```python
from build123d import *

# Parameters (mm, degrees)
SKETCH1_R               = 5
SKETCH1_W               = 4.1
SKETCH1_H               = 4.1
BOSS_EXTRUDE1_DEPTH     = 6
SKETCH1_3_R             = 8
SKETCH1_3_R_2           = 5
BOSS_EXTRUDE2_DEPTH     = 3
SKETCH1_6_R             = 8
SKETCH1_6_R_2           = 5
CUT_EXTRUDE_THIN1_DEPTH = 1.5


with BuildPart() as part:
    # Sketch1 → Boss-Extrude1 (new, symmetric)
    with BuildSketch(Plane.XY):
        Circle(SKETCH1_R)
        Rectangle(SKETCH1_W, SKETCH1_H, mode=Mode.SUBTRACT)
    extrude(amount=BOSS_EXTRUDE1_DEPTH, both=True)

    # Sketch1<3> → Boss-Extrude2 (add, symmetric)
    # profile 1 of 2: a face of its own
    with BuildSketch(Plane.XY):
        Circle(SKETCH1_3_R)
        Circle(SKETCH1_3_R_2, mode=Mode.SUBTRACT)
    # profile 2 of 2: a face of its own
    with BuildSketch(Plane.XY):
        Circle(SKETCH1_3_R)
        Circle(SKETCH1_3_R_2, mode=Mode.SUBTRACT)
    extrude(amount=BOSS_EXTRUDE2_DEPTH, both=True)

    # Sketch1<6> → Cut-Extrude-Thin1 (cut, symmetric)
    with BuildSketch(Plane.XY):
        Circle(SKETCH1_6_R)
        Circle(SKETCH1_6_R_2, mode=Mode.SUBTRACT)
    extrude(amount=CUT_EXTRUDE_THIN1_DEPTH, both=True, mode=Mode.SUBTRACT)


solid = part.part
```
The listing builds one solid part. Answer for the finished solid, in the listing's coordinates (mm). A direction names the side the tool comes from. Coordinates: 2 decimals unless noted, no trailing zeros. Loops run counter-clockwise (first coordinate to the right, second up) from the corner with the lowest first, then second, coordinate; pieces in that order, holes last. Notation, with made-up numbers: (-35, 16.25) - (-14, 16.25) arc R26 cw to (-14, 52.25) - close; hole circle Ø7 at (15.25, -28). An arc over 180 degrees is marked (long way). Write item = value, one per line.
1) Section D-D (x = 2.5) is taken. Determine the outline of the cut face in (y, z), plus the area to 3 significant figures.
Responses:
outline = (-7.6, -3) - (-4.33, -3) - (-4.33, -6) - (4.33, -6) - (4.33, -3) - (7.6, -3) - (7.6, -1.5) - (4.33, -1.5) - (4.33, 1.5) - (7.6, 1.5) - (7.6, 3) - (4.33, 3) - (4.33, 6) - (-4.33, 6) - (-4.33, 3) - (-7.6, 3) - (-7.6, 1.5) - (-4.33, 1.5) - (-4.33, -1.5) - (-7.6, -1.5) - close
area = 124 mm^2
2) Determine the mould class of faces 6 (the face through (0, 2.05, 0)), 7 (the face through (-1.08, -4.88, 4.52)), 8 (the face through (5.2, 0.1, -3)) for opening direction X: pulls with the +X half, pulls with the -X half, needs draft (parallel to the pull), parting line crosses it, or undercut.
Responses:
face_6 = undercut
face_7 = parting line crosses it
face_8 = needs draft
3) Which of the six approach directions +Z, -Z, +X, -X, +Y, -Y give full straight-line access (tool end or side, diameter ignored) to faces 1 (the face through (5.2, 0.1, 3)), 2 (the face through (-1.08, -4.88, -4.48)), 3 (the face through (-0.1, -2.2, -6)), 4 (the face through (5.2, 0.1, 1.5)), 5 (the face through (-2.05, 0, 0))?
Responses:
face_1 = +Z
face_2 = -Z
face_3 = -Z, +X, -X, +Y, -Y
face_4 = none
face_5 = +Z, -Z
4) Find the intervals of material crossed by line 1 along Z through (x, y) = (4.75, 1.75); line 2 along Y through (x, z) = (0, 3.5); line 3 along X through (y, z) = (-0.25, 2), in increasing order.
Responses:
line_1 = -3 to -1.5, 1.5 to 3
line_2 = -5 to -2.05, 2.05 to 5
line_3 = -8 to -2.05, 2.05 to 8
5) Section A-A (y = 0) is taken. Determine the outline of the cut face in (x, z), plus the area to 3 significant figures.
Responses:
outline = (-8, -3) - (-5, -3) - (-5, -6) - (-2.05, -6) - (-2.05, 6) - (-5, 6) - (-5, 3) - (-8, 3) - (-8, 1.5) - (-5, 1.5) - (-5, -1.5) - (-8, -1.5) - close; (2.05, -6) - (5, -6) - (5, -3) - (8, -3) - (8, -1.5) - (5, -1.5) - (5, 1.5) - (8, 1.5) - (8, 3) - (5, 3) - (5, 6) - (2.05, 6) - close
area = 88.8 mm^2
6) Each of these flat-tipped pins is pushed along its axis until it touches: P1, Ø1.2, axis at y = -0.5, z = 1, coming from the +X side; P2, Ø1.5, axis at y = 2, z = -3, coming from the -X side; P3, Ø2, axis at x = 1.5, z = -1.5, coming from the +Y side. Where does it stop, or does it pass through?
Responses:
P1 = 8
P2 = -7.9
P3 = 7.98
7) Section B-B (z = 2) is taken. Determine the outline of the cut face in (x, y), plus the area to 3 significant figures.
Responses:
outline = circle Ø16 at (0, 0); hole (-2.05, -2.05) - (2.05, -2.05) - (2.05, 2.05) - (-2.05, 2.05) - close
area = 184 mm^2
